from build123d import *

# Parameters (mm, degrees)
AUFSATZ_LINEAR_AUSTRAGEN1_DEPTH = 1
SKIZZE2_W                       = 16
SKIZZE2_H                       = 10
SKIZZE2_W_2                     = 15.5
AUFSATZ_LINEAR_AUSTRAGEN2_DEPTH = 1
SKIZZE4_W                       = 93.5
SKIZZE4_H                       = 1
SKIZZE4_W_2                     = 1
SKIZZE4_H_2                     = 67
AUFSATZ_LINEAR_AUSTRAGEN5_DEPTH = 2
VERRUNDUNG1_R                   = 1.3
VERRUNDUNG2_R                   = 1.3
VERRUNDUNG3_R                   = 1.3
VERRUNDUNG4_R                   = 1.3
VERRUNDUNG5_R                   = 1.3
VERRUNDUNG6_R                   = 1.3
VERRUNDUNG7_R                   = 1.3
VERRUNDUNG8_R                   = 1.3
VERRUNDUNG9_R                   = 1.3
VERRUNDUNG10_R                  = 1.3
VERRUNDUNG11_R                  = 1.3
VERRUNDUNG12_R                  = 1.3
VERRUNDUNG13_R                  = 1.3


with BuildPart() as part:
    # Skizze1 → Aufsatz-Linear austragen1 (new body)
    with BuildSketch(Plane.XY):
        Polygon((-31, -15.187500578), (-31, 32.5), (-21, 32.5), (-21, 5), (21, 5), (21, 32.5), (31, 32.5), (31, -34.5), (21, -34.5), (21, -5), (-21, -5), (-21, -34.5), (-31, -34.5), align=None)
    extrude(amount=AUFSATZ_LINEAR_AUSTRAGEN1_DEPTH)

    # Skizze2 → Aufsatz-Linear austragen2 (add)
    with BuildSketch(Plane(origin=(0, 0, 0), x_dir=(-1, 0, 0), z_dir=(0, 0, -1))):
        with Locations((39, 0)):
            Rectangle(SKIZZE2_W, SKIZZE2_H)
        with Locations((-38.75, 0)):
            Rectangle(SKIZZE2_W_2, SKIZZE2_H)
    extrude(amount=-AUFSATZ_LINEAR_AUSTRAGEN2_DEPTH)

    # Skizze4 → Aufsatz-Linear austragen5 (add)
    with BuildSketch(Plane(origin=(0, 0, 0), x_dir=(-1, 0, 0), z_dir=(0, 0, -1))):
        with Locations((0.25, 1.8)):
            Rectangle(SKIZZE4_W, SKIZZE4_H)
        with Locations((0.25, -1.8)):
            Rectangle(SKIZZE4_W, SKIZZE4_H)
        with Locations((-27.8, -1)):
            Rectangle(SKIZZE4_W_2, SKIZZE4_H_2)
        with Locations((-24.2, -1)):
            Rectangle(SKIZZE4_W_2, SKIZZE4_H_2)
        with Locations((24.2, -1)):
            Rectangle(SKIZZE4_W_2, SKIZZE4_H_2)
        with Locations((27.8, -1)):
            Rectangle(SKIZZE4_W_2, SKIZZE4_H_2)
    extrude(amount=AUFSATZ_LINEAR_AUSTRAGEN5_DEPTH)

    # Verrundung1
    verrundung1_edges = [part.edges().sort_by_distance(p)[0] for p in [
        (24.7, 17.4, 0),
    ]]
    fillet(verrundung1_edges, radius=VERRUNDUNG1_R)

    # Verrundung2
    verrundung2_edges = [part.edges().sort_by_distance(p)[0] for p in [
        (27.3, 17.4, 0),
    ]]
    fillet(verrundung2_edges, radius=VERRUNDUNG2_R - 0.0001)  # a hair under: the kernel refuses the full size

    # Verrundung3
    verrundung3_edges = [part.edges().sort_by_distance(p)[0] for p in [
        (37.4, 1.3, 0),
        (26, 1.3, 0),
        (0, 1.3, 0),
        (-26, 1.3, 0),
        (-37.65, 1.3, 0),
    ]]
    fillet(verrundung3_edges, radius=VERRUNDUNG3_R)

    # Verrundung4
    verrundung4_edges = [part.edges().sort_by_distance(p)[0] for p in [
        (37.4, -1.3, 0),
        (26, -1.3, 0),
        (0, -1.3, 0),
        (-26, -1.3, 0),
        (-37.65, -1.3, 0),
    ]]
    fillet(verrundung4_edges, radius=VERRUNDUNG4_R - 0.0001)  # a hair under: the kernel refuses the full size

    # Verrundung5
    verrundung5_edges = [part.edges().sort_by_distance(p)[0] for p in [
        (24.7, 2.3, -1.65),
        (27.3, 2.3, -1.64995),
        (26.919268105, 2.3, -0.380731895),
        (25.080761184, 2.3, -0.380761184),
    ]]
    fillet(verrundung5_edges, radius=VERRUNDUNG5_R - 0.0001)  # a hair under: the kernel refuses the full size

    # Verrundung6
    verrundung6_edges = [part.edges().sort_by_distance(p)[0] for p in [
        (24.7, 1.3, -1.65),
        (24.7, -1.3, -1.64995),
        (28.3, 1.3, -1.65),
        (28.3, -1.3, -1.64995),
        (24.7, -0.919268105, -0.380731895),
        (24.7, 0.919238816, -0.380761184),
        (28.3, 0.919238816, -0.380761184),
        (28.3, -0.919268105, -0.380731895),
    ]]
    fillet(verrundung6_edges, radius=VERRUNDUNG6_R - 0.0001)  # a hair under: the kernel refuses the full size

    # Verrundung7
    verrundung7_edges = [part.edges().sort_by_distance(p)[0] for p in [
        (23.7, -1.3, -1.64995),
        (23.7, 1.3, -1.65),
        (27.3, -1.3, -1.64995),
        (27.3, 1.3, -1.65),
        (23.7, 0.919238816, -0.380761184),
        (23.7, -0.919268105, -0.380731895),
        (27.3, -0.919268105, -0.380731895),
        (27.3, 0.919238816, -0.380761184),
    ]]
    fillet(verrundung7_edges, radius=VERRUNDUNG7_R - 0.0001)  # a hair under: the kernel refuses the full size

    # Verrundung8
    verrundung8_edges = [part.edges().sort_by_distance(p)[0] for p in [
        (27.3, -18.4, 0),
        (24.7, -18.4, 0),
    ]]
    fillet(verrundung8_edges, radius=VERRUNDUNG8_R - 0.0001)  # a hair under: the kernel refuses the full size

    # Verrundung9
    verrundung9_edges = [part.edges().sort_by_distance(p)[0] for p in [
        (27.3, -2.3, -1.64995),
        (24.7, -2.3, -1.64995),
        (25.080731895, -2.3, -0.380731895),
        (26.919268105, -2.3, -0.380731895),
    ]]
    fillet(verrundung9_edges, radius=VERRUNDUNG9_R - 0.0001)  # a hair under: the kernel refuses the full size

    # Verrundung10
    verrundung10_edges = [part.edges().sort_by_distance(p)[0] for p in [
        (-24.7, -1.3, -1.64995),
        (-24.7, -0.919268105, -0.380731895),
        (-24.7, 1.3, -1.65),
        (-28.3, -1.3, -1.64995),
        (-28.3, 1.3, -1.65),
        (-24.7, 0.919238816, -0.380761184),
        (-24.7, -18.4, 0),
        (-24.7, 17.4, 0),
        (-28.3, -0.919268105, -0.380731895),
        (-28.3, 0.919238816, -0.380761184),
    ]]
    fillet(verrundung10_edges, radius=VERRUNDUNG10_R - 0.0001)  # a hair under: the kernel refuses the full size

    # Verrundung11
    verrundung11_edges = [part.edges().sort_by_distance(p)[0] for p in [
        (-23.7, 1.3, -1.65),
        (-23.7, -1.3, -1.64995),
        (-27.3, 1.3, -1.65),
        (-27.3, -1.3, -1.64995),
        (-27.3, -18.4, 0),
        (-23.7, -0.919268105, -0.380731895),
        (-23.7, 0.919238816, -0.380761184),
        (-27.3, -0.919268105, -0.380731895),
        (-27.3, 0.919238816, -0.380761184),
        (-27.3, 17.4, 0),
    ]]
    fillet(verrundung11_edges, radius=VERRUNDUNG11_R - 0.0001)  # a hair under: the kernel refuses the full size

    # Verrundung12
    verrundung12_edges = [part.edges().sort_by_distance(p)[0] for p in [
        (-24.7, -2.3, -1.64995),
        (-27.3, -2.3, -1.64995),
        (-25.080731895, -2.3, -0.380731895),
        (-26.919268105, -2.3, -0.380731895),
    ]]
    fillet(verrundung12_edges, radius=VERRUNDUNG12_R - 0.0001)  # a hair under: the kernel refuses the full size

    # Verrundung13
    verrundung13_edges = [part.edges().sort_by_distance(p)[0] for p in [
        (-27.3, 2.3, -1.64995),
        (-24.7, 2.3, -1.64995),
        (-25.080731895, 2.3, -0.380731895),
        (-26.919268105, 2.3, -0.380731895),
    ]]
    fillet(verrundung13_edges, radius=VERRUNDUNG13_R - 0.0001)  # a hair under: the kernel refuses the full size


solid = part.part
Work out the finished part from the listing and answer in its coordinate system (mm). A direction names the side the tool comes from. Give positions to 0.01 mm unless a question says otherwise; leave off trailing zeros. Order: outer loops, then holes, each group sorted by start corner. A loop starts at its lowest first (then second) coordinate and runs counter-clockwise, first axis right, second up. Notation, with made-up numbers: (-7.5, -39) -> (28.5, -39) arc R21 cw to (28.5, -21) -> close; hole circle Ø4 at (14.25, -38). An arc over 180 degrees is marked (long way). Answer as a JSON object with one key per item and string values. Group by question number.
1. A tool of negligible diameter and unlimited length cuts with its end or side. For faces 1 (the flat face through (30.7, 13, 0)), 2 (the flat face through (-28.3, 17, -1)), 3 (the flat face through (-23.7, -19, -1)), 4 (the flat face through (38, -2.3, -1)), 5 (the flat face through (4, 4, 0)), from which of +Z, -Z, +X, -X, +Y, -Y can it reach the whole face along a straight path? Write none if from no direction.
2. Flat-ended cylindrical pins translate along their axes: pin 1 Ø1.6 at (y, z) = (-22.5, -1) entering from +X; pin 2 Ø1.5 at (x, z) = (-8, -0.5) entering from +Y; pin 3 Ø1.1 at (y, z) = (23.5, 0.5) entering from -X. Find the tip coordinate at first contact, or state that the pin passes through.
3. Consider line 1 along X through (y, z) = (-24, -1.6); line 2 along X through (y, z) = (6.5, -0.35); line 3 along X through (y, z) = (-24.5, 0.75). Determine where each line is inside the solid, lowest interval first. Write a range as [from, to].
4. Section C-C on z = 0.5 is taken. Determine the outline of the cut face in (x, y), plus the area to 4 significant figures.
Result sheet:
{
 "1": {"face 1": "-Z, +X, +Y", "face 2": "-Z, -X, +Y", "face 3": "-Z, -Y", "face 4": "-Z, +X, -Y", "face 5": "-Z, +Y"},
 "2": {"pin 1": "stops at x = 28.3", "pin 2": "stops at y = 5", "pin 3": "stops at x = -31"},
 "3": {"line 1": "x = [-28.3, -27.3], [-24.7, -23.7], [23.7, 24.7], [27.3, 28.3]", "line 2": "x = [-28.3, -26.89], [-25.11, -23.7], [23.7, 25.11], [26.89, 28.3]", "line 3": "x = [-31, -21], [21, 31]"},
 "4": {"outline": "(-47, -5) -> (-31, -5) -> (-31, -34.5) -> (-21, -34.5) -> (-21, -5) -> (21, -5) -> (21, -34.5) -> (31, -34.5) -> (31, -5) -> (46.5, -5) -> (46.5, 5) -> (31, 5) -> (31, 32.5) -> (21, 32.5) -> (21, 5) -> (-21, 5) -> (-21, 32.5) -> (-31, 32.5) -> (-31, 5) -> (-47, 5) -> close", "area": "2,075 mm^2"}
}
